Could you check a few things on this drawing? It's one solid part, dimensions in mm from its lowest x, y, z. A direction names the side the tool comes from. Give positions to 0.01 mm unless a question says otherwise; leave off trailing zeros. Loops run counter-clockwise (first coordinate to the right, second up) from the corner with the lowest first, then second, coordinate; pieces in that order, holes last.
1. Thinking about a two-plate mould opening in X: for the marked faces 4, 5 and 6, which applies, +X half, -X half, draft (parallel to the pull), parting line (faces both ways), or undercut?
2. For P1, Ø6, axis at y = 16, z = 4.5, coming from the -X side; P2, Ø10, axis at x = 41.5, y = 17, coming from the +Z side; P3, Ø5, axis at y = 7, z = 5, coming from the +X side, each with a flat end and sliding along its axis, tell me the tip position at first contact or that it passes through.
3. Imagine slicing it at A-A (y = 2.5). List the corners of the cut face in (x, z) for me (1 decimal).
4. Imagine slicing it at C-C (y = 10). List the corners of the cut face in (x, z) for me.
5. Imagine slicing it at D-D (z = 9). List the corners of the cut face in (x, y) for me.
6. For the marked faces 1, 2 and 3, which set-ups out of +Z, -Z, +X, -X, +Y, -Y let a thin tool reach every point of the face, with its end or its side?
7. Imagine slicing it at B-B (x = 70). List the corners of the cut face in (y, z) for me, plus the area to 3 significant figures.
8. I need wall thicknesses on line 1 along Y through (x, z) = (61, 4); line 2 along X through (y, z) = (12.5, 8.5); line 3 along Z through (x, y) = (32, 7.5). Which ranges of each line are inside material? Lowest first, please.
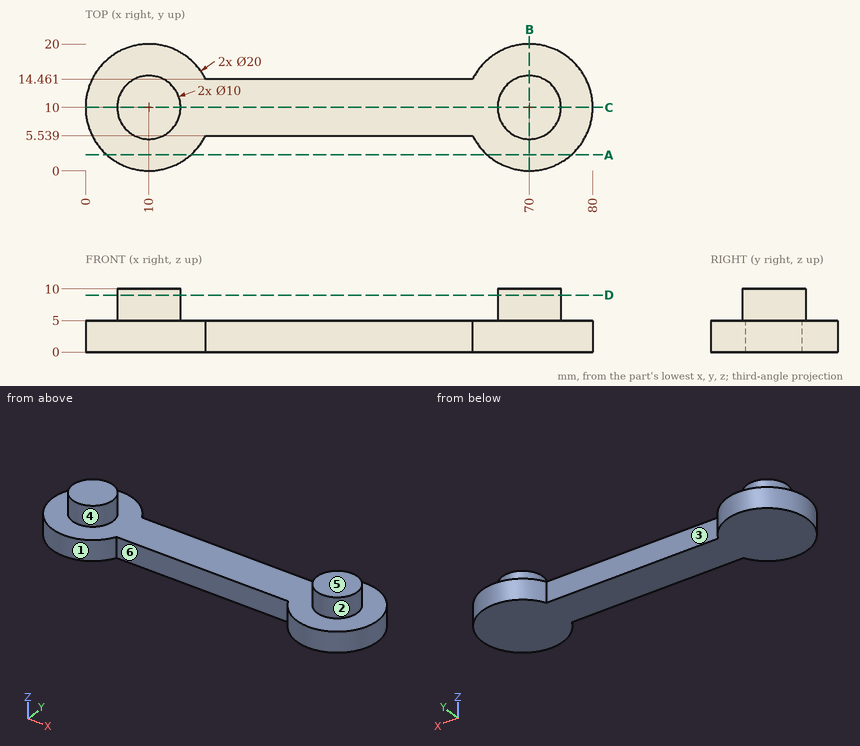
Derived:
1. face 4: undercut
1. face 5: draft
1. face 6: undercut
2. P1: stops at x = 0.46
2. P2: stops at z = 5
2. P3: stops at x = 79.99
3. outline: (3.4, 0) - (16.6, 0) - (16.6, 5) - (3.4, 5) - close; (63.4, 0) - (76.6, 0) - (76.6, 5) - (63.4, 5) - close
4. outline: (0, 0) - (80, 0) - (80, 5) - (75, 5) - (75, 10) - (65, 10) - (65, 5) - (15, 5) - (15, 10) - (5, 10) - (5, 5) - (0, 5) - close
5. outline: circle Ø10 at (10, 10); circle Ø10 at (70, 10)
6. face 1: +Z, -Z
6. face 2: +Z
6. face 3: +Z, -Z, +Y
7. outline: (0, 0) - (20, 0) - (20, 5) - (15, 5) - (15, 10) - (5, 10) - (5, 5) - (0, 5) - close
7. area: 150 mm2
8. line 1: y = 5.54 to 14.46
8. line 2: x = 5.67 to 14.33, 65.67 to 74.33
8. line 3: z = 0 to 5
